from build123d import *

# Parameters (mm, degrees)
SKETCH1_W               = 320
SKETCH1_H               = 200
SKETCH1_W_2             = 280
SKETCH1_H_2             = 160
BOSS_EXTRUDE1_DEPTH     = 20
SKETCH2_W               = 150
SKETCH2_H               = 200
CUT_EXTRUDE1_DEPTH      = 20
SKETCH3_W               = 20
SKETCH3_H               = 20
BOSS_EXTRUDE2_DEPTH     = 60
SKETCH4_W               = 12
SKETCH4_H               = 16
CUT_EXTRUDE2_DEPTH      = 20
SKETCH5_W               = 12
SKETCH5_H               = 12
CUT_EXTRUDE3_DEPTH      = 22
CUT_EXTRUDE5_DEPTH      = 275.40845468
CUT_EXTRUDE5_DEPTH_BACK = 275.40845468
SKETCH8_R               = 3
SKETCH10_R              = 3
CUT_EXTRUDE6_DEPTH      = 30
SKETCH11_W              = 14
SKETCH11_H              = 50
CUT_EXTRUDE7_DEPTH      = 6
SKETCH12_R              = 3
CUT_EXTRUDE8_DEPTH      = 26
SKETCH13_R              = 3
CUT_EXTRUDE9_DEPTH      = 26


with BuildPart() as part:
    # Sketch1 → Boss-Extrude1 (new body)
    with BuildSketch(Plane(origin=(0, 0, 0), x_dir=(1, 0, 0), z_dir=(0, 1, 0))):
        with Locations((160, 100)):
            Rectangle(SKETCH1_W, SKETCH1_H)
        with Locations((160, 100)):
            Rectangle(SKETCH1_W_2, SKETCH1_H_2, mode=Mode.SUBTRACT)
    extrude(amount=BOSS_EXTRUDE1_DEPTH)

    # Sketch2 → Cut-Extrude1 (cut)
    with BuildSketch(Plane(origin=(0, 20, 0), x_dir=(1, 0, 0), z_dir=(0, 1, 0))):
        with Locations((245, 100)):
            Rectangle(SKETCH2_W, SKETCH2_H)
    extrude(amount=-CUT_EXTRUDE1_DEPTH, mode=Mode.SUBTRACT)

    # Sketch3 → Boss-Extrude2 (add)
    with BuildSketch(Plane(origin=(0, 20, 0), x_dir=(1, 0, 0), z_dir=(0, 1, 0))):
        with Locations((10, 10)):
            Rectangle(SKETCH3_W, SKETCH3_H)
        with Locations((10, 190)):
            Rectangle(SKETCH3_W, SKETCH3_H)
    extrude(amount=BOSS_EXTRUDE2_DEPTH)

    # Sketch4 → Cut-Extrude2 (cut)
    with BuildSketch(Plane(origin=(0, 80, 0), x_dir=(1, 0, 0), z_dir=(0, 1, 0))):
        with Locations((10, 10)):
            Rectangle(SKETCH4_W, SKETCH4_H)
        with Locations((10, 190)):
            Rectangle(SKETCH4_W, SKETCH4_H)
    extrude(amount=-CUT_EXTRUDE2_DEPTH, mode=Mode.SUBTRACT)

    # Sketch5 → Cut-Extrude3 (cut)
    with BuildSketch(Plane(origin=(170, 0, 0), x_dir=(0, 0, -1), z_dir=(1, 0, 0))):
        with Locations((10, 10)):
            Rectangle(SKETCH5_W, SKETCH5_H)
        with Locations((190, 10)):
            Rectangle(SKETCH5_W, SKETCH5_H)
    extrude(amount=-CUT_EXTRUDE3_DEPTH, mode=Mode.SUBTRACT)

    # Sketch8 → Cut-Extrude5 (cut, two sides: drawn at the far end of the back side and taken through both)
    with BuildSketch(Plane(origin=(0, 0, -200), x_dir=(-1, 0, 0), z_dir=(0, 0, -1)).offset(-CUT_EXTRUDE5_DEPTH_BACK)):
        with Locations((-30, 10)):
            Circle(SKETCH8_R)
        with Locations((-160, 10)):
            Circle(SKETCH8_R)
        with Locations((-70, 10)):
            Circle(SKETCH8_R)
        with Locations((-130, 10)):
            Circle(SKETCH8_R)
    extrude(amount=CUT_EXTRUDE5_DEPTH + CUT_EXTRUDE5_DEPTH_BACK, mode=Mode.SUBTRACT)

    # Sketch10 → Cut-Extrude6 (cut)
    with BuildSketch(Plane.XZ):
        with Locations(Location((142.5, -10, 0), (0, 0, 270))):
            Circle(SKETCH10_R)
        with Locations(Location((95, -10, 0), (0, 0, 270))):
            Circle(SKETCH10_R)
        with Locations(Location((10, -100, 0), (0, 0, 270))):
            Circle(SKETCH10_R)
        with Locations(Location((142.5, -190, 0), (0, 0, 270))):
            Circle(SKETCH10_R)
        with Locations(Location((95, -190, 0), (0, 0, 270))):
            Circle(SKETCH10_R)
    extrude(amount=-CUT_EXTRUDE6_DEPTH, mode=Mode.SUBTRACT)

    # Sketch11 → Cut-Extrude7 (cut)
    with BuildSketch(Plane(origin=(20, 0, 0), x_dir=(0, 0, -1), z_dir=(1, 0, 0))):
        with Locations((7, 55)):
            Rectangle(SKETCH11_W, SKETCH11_H)
    extrude(amount=-CUT_EXTRUDE7_DEPTH, mode=Mode.SUBTRACT)

    # Sketch12 → Cut-Extrude8 (cut)
    with BuildSketch(Plane.ZY):
        with Locations((-133, 10)):
            Circle(SKETCH12_R)
        with Locations((-67, 10)):
            Circle(SKETCH12_R)
    extrude(amount=-CUT_EXTRUDE8_DEPTH, mode=Mode.SUBTRACT)

    # Sketch13 → Cut-Extrude9 (cut)
    with BuildSketch(Plane.ZY):
        with Locations((-191.8, 70)):
            Circle(SKETCH13_R)
        with Locations((-8.2, 70)):
            Circle(SKETCH13_R)
    extrude(amount=-CUT_EXTRUDE9_DEPTH, mode=Mode.SUBTRACT)


solid = part.part
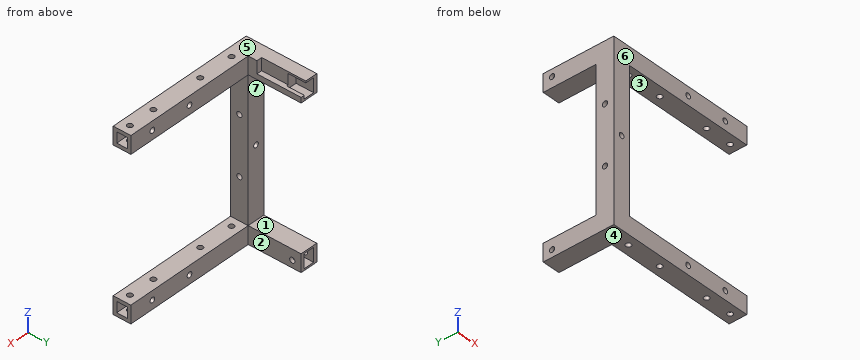
Build history of the part. All positions in model axes, mm. Face numbers are marked on the shaded views. A direction names the side the tool comes from. Round coordinates to 2 decimals unless told otherwise and drop trailing zeros. Loops run counter-clockwise (first coordinate to the right, second up) from the corner with the lowest first, then second, coordinate; pieces in that order, holes last. Notation, with made-up numbers: (66.5, 33) -> (84.5, 33) arc R18 cw to (84.5, 53) -> close; hole circle Ø3 at (89.25, 78.5). An arc over 180 degrees is marked (long way). Use CSV: the item, a comma, the result in double quotes. Start each with the question number.
Q1. Saw through at C-C on x = 10. Give the cut face in (y, z), and give its area (3 significant figures).
Q2. Saw through at A-A on x = 112. Give the cut face in (y, z), and give its area (3 significant figures).
Q3. Which spindle directions (+Z, -Z, +X, -X, +Y, -Y) get a long thin tool onto all of the face, cutting with end or side? Do the marked faces 1, 2 and 3. Say none if no direction does.
Q4. Saw through at D-D on y = 70. Count the separate pieces of the cut face and the enclosed holes in it, and give its area (3 significant figures).
Q5. Drill centre lines: L1, parallel to X at y = 10, z = -3.15; L2, parallel to Z at x = 56, y = 9.5; L3, parallel to Y at x = 30, z = -12.5. Where is each one in solid material? Low to high.
Q6. Flat gauge pins, fed straight in: pin 1 Ø6 at (y, z) = (37.5, -176) entering from +X; pin 2 Ø16 at (x, z) = (11.5, -134) entering from +Y; pin 3 Ø6 at (y, z) = (61, -5) entering from +X; pin 4 Ø15.5 at (y, z) = (61, -8) entering from +X. Where does each tip first touch, or does it go through?
Q7. Mould opens along Z. For the marked faces 4, 5, 6 and 7 say: +Z half, -Z half, draft (parallel to the pull), parting line (faces both ways), or undercut.
Solutions:
1,outline,"(0, -200) -> (80, -200) -> (80, -198) -> (60, -198) -> (60, -182) -> (80, -182) -> (80, -180) -> (20, -180) -> (20, -103) -> (0, -103) -> close; (0, -97) -> (20, -97) -> (20, -20) -> (80, -20) -> (80, -18) -> (60, -18) -> (60, -2) -> (80, -2) -> (80, 0) -> (0, 0) -> close; hole circle Ø6 at (10, -133); hole circle Ø6 at (10, -67)"
1,area,"5,580 mm^2"
2,outline,"(0, -200) -> (20, -200) -> (20, -180) -> (0, -180) -> close; (0, -20) -> (20, -20) -> (20, 0) -> (0, 0) -> close"
2,area,"800 mm^2"
3,face 1,"+X, -X, +Y"
3,face 2,"+Z, -Z, +X, +Y"
3,face 3,"+X, +Y, -Y"
4,separate pieces,"4"
4,enclosed holes,"0"
4,area,"284 mm^2"
5,L1,"x = 0 to 27, 33 to 67, 73 to 127, 133 to 157, 163 to 170"
5,L2,"z = -200 to -180, -20 to 0"
5,L3,"y = 0 to 7, 13 to 20"
6,pin 1,"passes through"
6,pin 2,"stops at y = 20"
6,pin 3,"stops at x = 14"
6,pin 4,"stops at x = 20"
7,face 4,"-Z half"
7,face 5,"+Z half"
7,face 6,"draft"
7,face 7,"undercut"
